Could you check a few things on this model? Use its own coordinates, in mm. Give positions to 0.01 mm unless a question says otherwise; leave off trailing zeros. Loops run counter-clockwise (first coordinate to the right, second up) from the corner with the lowest first, then second, coordinate; pieces in that order, holes last. Notation, with made-up numbers: M 72,10.25 L 107,10.25 A15 cw 107,15.25 Z; hole C -32.75,52 d6. An arc over 180 degrees is marked long. Answer in a Markdown table with one row per item. Add a question column.
Autodesk Inventor part; units mm, degrees
ref_plane "YZ Plane" through (0, 0, 0) normal (1, 0, 0) x (0, 1, 0)
ref_plane "XZ Plane" through (0, 0, 0) normal (0, 1, 0) x (-1, 0, 0)
ref_plane "XY Plane" through (0, 0, 0) normal (0, 0, 1) x (1, 0, 0)
sketch "Sketch1" plane through (0, 0, 0) normal (0, 0, 1) x (1, 0, 0)
  line L0 (-90, 21.5) -> (0, 21.5)
  line L1 (0, 21.5) -> (0, -21.5)
  line L2 (0, -21.5) -> (-90, -21.5)
  line L3 (-90, -21.5) -> (-90, 21.5)
  line L4 (-90, 21.5) -> (-142, 21.5)
  line L5 (-142, 21.5) -> (-142, -21.5)
  line L6 (-142, -21.5) -> (-90, -21.5)
  line L7 (-90, -21.5) -> (-90, 21.5)
  line L8 (-96, 21.5) -> (-96, -21.5)
  line L9 (-136, 21.5) -> (-136, -21.5)
  line L10 (-172, 39.3338) -> (-172, -34.4361) construction
  line L11 (-172, 12.5) -> (-192, 12.5)
  line L12 (-192, 12.5) -> (-192, -12.5)
  line L13 (-192, -12.5) -> (-172, -12.5)
  line L14 (-172, -12.5) -> (-172, 12.5)
  line L15 (-237.0195, 0) -> (143.1564, 0) construction
  line L16 (0, 148.4042) -> (0, -100.7046) construction
  line L17 (-172, 12.5) -> (-142, 21.5)
  line L18 (-172, -12.5) -> (-142, -21.5)
  line L19 (-20, 21.5) -> (-20, -21.5)
  line L20 (0, 10) -> (15, 10)
  line L21 (15, 10) -> (15, -10)
  line L22 (15, -10) -> (0, -10)
  line L23 (0, -10) -> (0, 10)
  line L24 (-63.7943, -15.2321) -> (-63.7943, 15.4179)
  line L25 (-63.7943, 15.4179) -> (-44.6843, 15.4179)
  line L26 (-44.6843, 15.4179) -> (-44.6843, -15.2321)
  line L27 (-44.6843, -15.2321) -> (-63.7943, -15.2321)
  line L28 (-86.4422, 19.0102) -> (-68.4422, 19.0102)
  line L29 (-68.4422, 19.0102) -> (-68.4422, -18.9898)
  line L30 (-68.4422, -18.9898) -> (-86.4422, -18.9898)
  line L31 (-86.4422, -18.9898) -> (-86.4422, 19.0102)
  line L32 (-41.3198, 14.7798) -> (-22.3198, 14.7798)
  line L33 (-22.3198, 14.7798) -> (-22.3198, -4.2202)
  line L34 (-22.3198, -4.2202) -> (-41.3198, -4.2202)
  line L35 (-41.3198, -4.2202) -> (-41.3198, 14.7798)
  line L36 (-41.3198, -7.7055) -> (-24.4109, -7.7055)
  line L37 (-24.4109, -7.7055) -> (-24.4109, -17)
  line L38 (-24.4109, -17) -> (-41.3198, -17)
  line L39 (-41.3198, -17) -> (-41.3198, -7.7055)
  point P0 (0, 0)
  point P1 (0, 0)
  point P2 (-172, 0)
  point P3 (15, 0)
  dimension "d0" = 90
  dimension "d1" = 43
  dimension "d2" = 6
  dimension "d3" = 6
  dimension "d5" = 40
  dimension "d6" = 30
  dimension "d7" = 20
  dimension "d8" = 25
  dimension "d23" = 20
  dimension "d34" = 15
  dimension "d35" = 20
  dimension "d36" = 19
  dimension "d37" = 19
  dimension "d38" = 30.65
  dimension "d39" = 19.11
  dimension "d40" = 38
  dimension "d41" = 18
extrude "Extrusion1" add sketch "Sketch1" along normal blind 0.2 contours L0 L19 L2 L3 | L3 L6 L8 L4 | L0 L1 L2 L19 | L8 L6 L9 L4 | L9 L6 L5 L4 | L20 L21 L22 L1 | L5 L18 L14 L17 | L14 L13 L12 L11 | L24 L25 L26 L27 | L28 L29 L30 L31 | L32 L33 L34 L35 | L36 L37 L38 L39
extrude "Extrusion3" add sketch "Sketch1" along normal blind 0.4 contours L0 L1 L2 L19 | L20 L21 L22 L1
extrude "Extrusion4" add sketch "Sketch1" along normal blind 0.4 contours L14 L13 L12 L11
equation "\"d19\" = material"
equation "\"d30\" = 2 * material"
equation "\"d32\" = 2 * material"
properties part number "BandSide"
Item 1: Suppose I cut it at B-B (y = 4). List the corners of the cut face in (x, z) for me.
Item 2: I need wall thicknesses on L1, parallel to X at y = 1.5, z = 0.3; L2, parallel to X at y = 14, z = 0.3; L3, parallel to Z at x = -76, y = 20.5. Which ranges of each line are inside material? Lowest first, please.
Item 3: For P1, Ø2, axis at x = -38, y = -1, coming from the +Z side, with a flat end and sliding along its axis, tell me the tip position at first contact or that it passes through.
Item 4: Suppose I cut it at D-D (x = -105.5). List the corners of the cut face in (y, z) for me, then the cut area to 3 significant figures.
Item 5: If we mould it in two halves opening along X, with no side actions, what happens to faces 1 (the face through (-90, 0, 0)), 2 (the face through (-97, 0, 0.2))? For each: +X half, -X half, draft (parallel to the pull), parting line (faces both ways), or undercut.
Item 6: Suppose I cut it at A-A (z = 0.3). List the corners of the cut face in (x, y) for me, then the cut area to 3 significant figures.
Item 7: Suppose I cut it at C-C (x = -166.5). List the corners of the cut face in (y, z) for me, then the cut area to 3 significant figures.
Values found:
| question | item | result |
|---|---|---|
| 1 | outline | M -192,0 L 15,0 L 15,0.4 L -20,0.4 L -20,0.2 L -172,0.2 L -172,0.4 L -192,0.4 Z |
| 2 | L1 | -192 to -172, -20 to 15 |
| 2 | L2 | -20 to 0 |
| 2 | L3 | 0 to 0.2 |
| 3 | P1 | z = 0.2 |
| 4 | outline | M -21.5,0 L 21.5,0 L 21.5,0.2 L -21.5,0.2 Z |
| 4 | area | 8.60 mm² |
| 5 | face 1 | draft |
| 5 | face 2 | undercut |
| 6 | outline | M -192,-12.5 L -172,-12.5 L -172,12.5 L -192,12.5 Z; M -20,-21.5 L 0,-21.5 L 0,-10 L 15,-10 L 15,10 L 0,10 L 0,21.5 L -20,21.5 Z |
| 6 | area | 1,660 mm² |
| 7 | outline | M -14.15,0 L 14.15,0 L 14.15,0.2 L -14.15,0.2 Z |
| 7 | area | 5.66 mm² |
